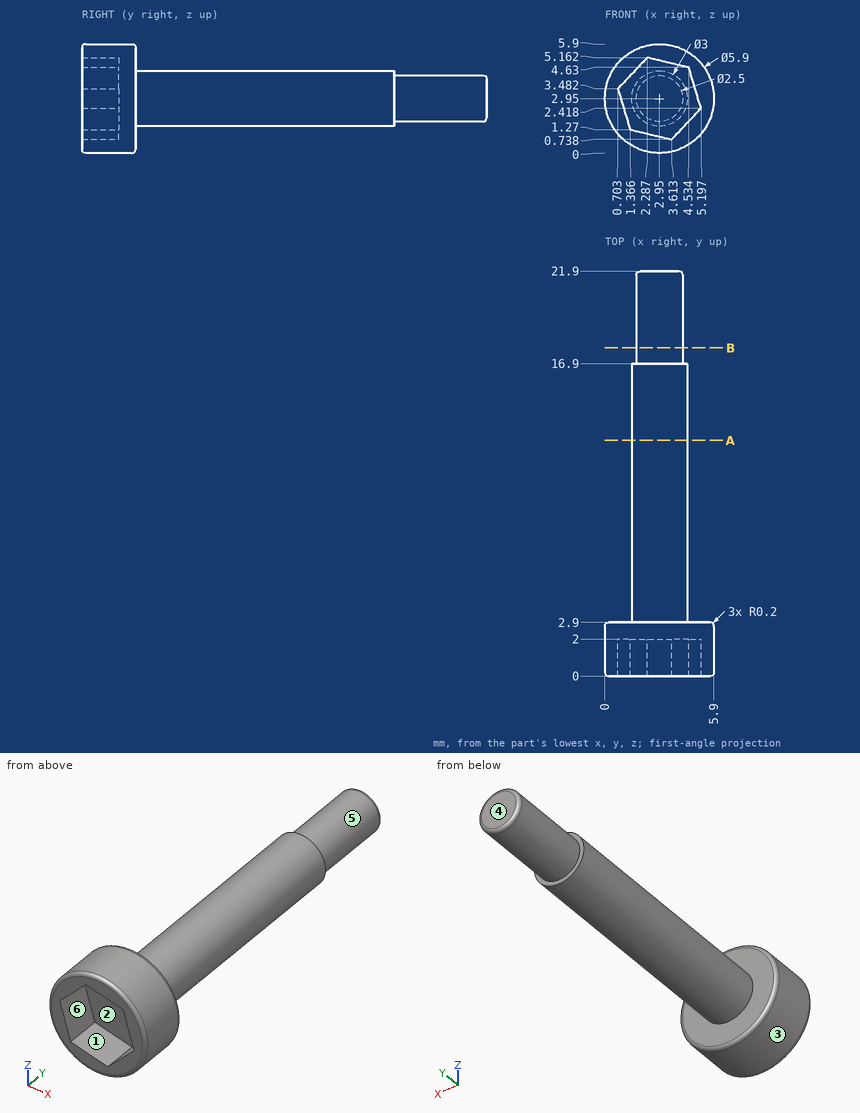
The drawing under review shows one solid part. Ordinate dimensions are in mm from its lowest x, y, z. A direction names the side the tool comes from. Give positions to 0.01 mm unless a question says otherwise; leave off trailing zeros. Write each loop counter-clockwise with the first axis right and the second up, starting at its lowest first coordinate (ties: lowest second). Pieces come first, ordered by that corner, then holes.
1. Add section A-A, the plane y = 12.75. Write out the cut boundary in (x, z).
2. Wall thickness on L1, parallel to Y at x = 5.4, z = 3.8; L2, parallel to Z at x = 4.35, y = 1.75 (1 decimal); L3, parallel to Y at x = 4, z = 1.2: over which ranges is each line inside the solid? List them lowest first.
3. Draft analysis for pull direction Z (two halves, no side actions). For the marked faces 1, 2, 3 and 4, state which applies: +Z half, -Z half, draft (parallel to the pull), parting line (faces both ways), or undercut.
4. Tool access review of the marked faces 5 and 6: name each direction out of +Z, -Z, +X, -X, +Y, -Y from which nothing blocks a thin tool from reaching the whole face with its end or side.
5. Add section B-B, the plane y = 17.75. Write out the cut boundary in (x, z).
6. For P1, Ø1, axis at x = 4.5, z = 4.5, coming from the +Y side; P2, Ø3, axis at x = 1, y = 19, coming from the -Z side; P3, Ø3, axis at x = 5, y = 10, coming from the -Z side (1 decimal), all flat-tipped, find the tip position at first contact; note any pin that passes through.
Worked answers:
1. outline: circle Ø3 at (2.95, 2.95)
2. L1: y = 0 to 2.9
2. L2: z = 0.4 to 1.5, 4.7 to 5.5
2. L3: y = 2 to 2.9
3. face 1: undercut
3. face 2: undercut
3. face 3: parting line
3. face 4: draft
4. face 5: +Y
4. face 6: -Y
5. outline: circle Ø2.5 at (2.95, 2.95)
6. P1: stops at y = 2.9
6. P2: stops at z = 1.78
6. P3: stops at z = 1.6
